Geometry: final body of the model. Coordinates: model frame, mm. Face numbers are marked on the shaded views. A direction names the side the tool comes from. Give positions to 0.01 mm unless a question says otherwise; leave off trailing zeros. Order: outer loops, then holes, each group sorted by start corner. A loop starts at its lowest first (then second) coordinate and runs counter-clockwise, first axis right, second up. Notation, with made-up numbers: (32.5, -37.75) - (37.5, -37.75) arc R27 cw to (37.5, -9.75) - close; hole circle Ø7 at (-5.5, -24.5). An arc over 180 degrees is marked (long way). Write item = value, one per line. Start each with the question number.
from build123d import *

# Parameters (mm, degrees)
SKETCH1_W                      = 15.5
SKETCH1_H                      = 19.5
SKETCH1_W_2                    = 9.9
SKETCH1_H_2                    = 13.9
BOSS_EXTRUDE1_DEPTH            = 4.05
SKETCH2_W                      = 19.5
SKETCH2_H                      = 9
SKETCH2_R                      = 1.5
BOSS_EXTRUDE2_DEPTH            = 2.8
CHAMFER1_SIZE                  = 2.5
FILLET1_R                      = 2
FILLET2_R                      = 0.5
CHAMFER2_SIZE                  = 0.5
CUT_EXTRUDE1_DEPTH             = 1.0000001
CUT_EXTRUDE1_DIRECTION_2_REACH = 17.5


with BuildPart() as part:
    # Sketch1 → Boss-Extrude1 (new body, symmetric)
    with BuildSketch(Plane(origin=(0, 0, 0), x_dir=(1, 0, 0), z_dir=(0, 1, 0))):
        Rectangle(SKETCH1_W, SKETCH1_H)
        Rectangle(SKETCH1_W_2, SKETCH1_H_2, mode=Mode.SUBTRACT)
    extrude(amount=BOSS_EXTRUDE1_DEPTH, both=True)

    # Sketch2 → Boss-Extrude2 (add)
    with BuildSketch(Plane.ZY.offset(7.75)):
        with Locations((0, -8.55)):
            Rectangle(SKETCH2_W, SKETCH2_H)
        with Locations((-5.25, -8.55)):
            Circle(SKETCH2_R, mode=Mode.SUBTRACT)
        with Locations((5.25, -8.55)):
            Circle(SKETCH2_R, mode=Mode.SUBTRACT)
    extrude(amount=-BOSS_EXTRUDE2_DEPTH)

    # Chamfer1
    chamfer1_edges = [part.edges().sort_by_distance(p)[0] for p in [
        (-4.95, -4.05, -8.35),
        (-4.95, -4.05, 8.35),
    ]]
    chamfer(chamfer1_edges, length=CHAMFER1_SIZE)

    # Fillet1
    fillet1_edges = [part.edges().sort_by_distance(p)[0] for p in [
        (-7.75, -4.5, -9.75),
        (7.75, 0, -9.75),
        (7.75, 0, 9.75),
        (-7.75, -4.5, 9.75),
    ]]
    fillet(fillet1_edges, radius=FILLET1_R)

    # Fillet2
    fillet2_edges = [part.edges().sort_by_distance(p)[0] for p in [
        (4.95, -4.05, 0),
        (1.25, -4.05, -6.95),
        (-4.95, 4.05, 0),
        (0, 4.05, 6.95),
        (4.95, 4.05, 0),
        (0, 4.05, -6.95),
        (-5.35, -13.05, -9.75),
        (-4.95, -9.8, 9.75),
        (-4.95, -13.05, 0),
        (-5.35, -13.05, 9.75),
        (1.65, -4.05, 9.75),
        (1.25, -4.05, 6.95),
        (-2.45, -4.05, 8.35),
        (-2.45, -4.05, -8.35),
        (-4.95, -9.8, -9.75),
        (-3.7, -5.3, -9.75),
        (-3.7, -5.3, -6.95),
        (-3.7, -5.3, 6.95),
        (-3.7, -5.3, 9.75),
        (1.65, -4.05, -9.75),
        (0, 4.05, -9.75),
        (7.75, -4.05, 0),
        (7.164213562, -4.05, 9.164213562),
        (7.164213562, -4.05, -9.164213562),
        (7.75, 4.05, 0),
        (-7.75, 4.05, 0),
        (0, 4.05, 9.75),
        (-7.164213562, 4.05, 9.164213562),
        (-7.164213562, 4.05, -9.164213562),
        (7.164213562, 4.05, 9.164213562),
        (7.164213562, 4.05, -9.164213562),
        (-7.75, -13.05, 0),
        (-7.164213562, -13.05, 9.164213562),
        (-7.164213562, -13.05, -9.164213562),
    ]]
    fillet(fillet2_edges, radius=FILLET2_R)

    # Chamfer2
    chamfer2_edges = [part.edges().sort_by_distance(p)[0] for p in [
        (-4.95, -8.55, 3.75),
        (-4.95, -8.55, -6.75),
    ]]
    chamfer(chamfer2_edges, length=CHAMFER2_SIZE)

    # Sketch3 → Cut-Extrude1 (cut)
    with BuildSketch(Plane.ZY.offset(7.75)):
        with BuildLine():
            Line((-3.5, 0.55), (3.5, 0.55))
            ThreePointArc((3.5, 0.55), (3.853553391, 0.403553391), (4, 0.05))
            Line((4, 0.05), (4, -2.22))
            ThreePointArc((4, -2.22), (3.853553391, -2.573553391), (3.5, -2.72))
            Line((3.5, -2.72), (-3.5, -2.72))
            ThreePointArc((-3.5, -2.72), (-3.853553391, -2.573553391), (-4, -2.22))
            Line((-4, -2.22), (-4, 0.05))
            ThreePointArc((-4, 0.05), (-3.853553391, 0.403553391), (-3.5, 0.55))
        make_face()
    extrude(amount=CUT_EXTRUDE1_DEPTH, mode=Mode.SUBTRACT)

    # Sketch3 → Cut-Extrude1 direction 2 (cut, up to next)
    with BuildSketch(Plane.ZY.offset(7.75), mode=Mode.PRIVATE) as cut_extrude1_direction_2_sk1:
        with BuildLine():
            Line((-3.5, 0.55), (3.5, 0.55))
            ThreePointArc((3.5, 0.55), (3.853553391, 0.403553391), (4, 0.05))
            Line((4, 0.05), (4, -2.22))
            ThreePointArc((4, -2.22), (3.853553391, -2.573553391), (3.5, -2.72))
            Line((3.5, -2.72), (-3.5, -2.72))
            ThreePointArc((-3.5, -2.72), (-3.853553391, -2.573553391), (-4, -2.22))
            Line((-4, -2.22), (-4, 0.05))
            ThreePointArc((-4, 0.05), (-3.853553391, 0.403553391), (-3.5, 0.55))
        make_face()
    cut_extrude1_direction_2_tool1 = extrude(cut_extrude1_direction_2_sk1.sketch, amount=-CUT_EXTRUDE1_DIRECTION_2_REACH, mode=Mode.PRIVATE) & part.part
    add(cut_extrude1_direction_2_tool1.solids().sort_by_distance((-7.75, -1.085, 0))[0], mode=Mode.SUBTRACT)


solid = part.part
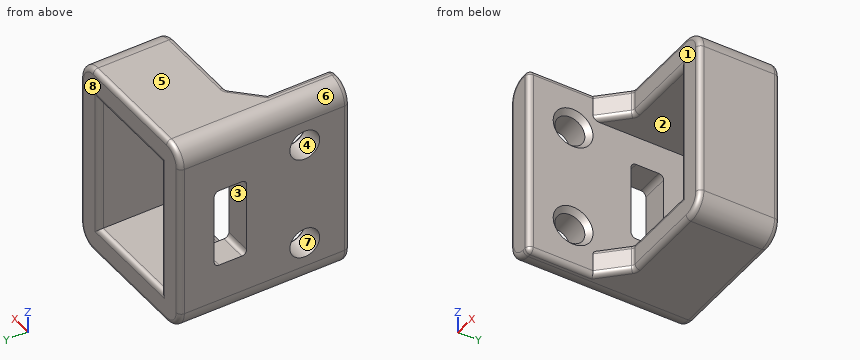
Q1. Pull-direction query (Y, two-part tool) for the marked faces 6, 7 and 8; classes: +Y half, -Y half, draft (parallel to the pull), parting line (faces both ways), or undercut.
Q2. Section B-B, the plane z = -0.5. Return the cut outline in (x, y).
Q3. Contact query for flat-ended pins moving along their axis: pin 1 (7.5 mm diameter, centred on x = 1.5, z = -3, fed in from -Y); pin 2 (0.7 mm diameter, centred on x = -7, y = -0.5, fed in from -Z). Output: stop coordinate, or through.
Q4. Material intervals for line 1 along Z through (x, y) = (1.5, 2.25); line 2 along Y through (x, z) = (-6.9, 5.25), sorted ascending. Write a range as from..to.
Q5. Section C-C, the plane y = -8.55. Return the cut outline in (x, z).
Q6. Set-up query: the marked faces 1, 2, 3, 4 and 5. Return all of +Z, -Z, +X, -X, +Y, -Y with unobstructed straight access to the full face (end or side cutting, diameter ignored); none if empty.
Q7. Section D-D, the plane z = 5.25. Return the cut outline in (x, y).
Q8. Section A-A, the plane x = 0.5. Return the cut outline in (y, z), then the cut area to 3 significant figures.
The answers:
q1.face_6 = draft
q1.face_7 = undercut
q1.face_8 = +Y half
q2.outline = (-7.75, -12.55) arc R0.5 ccw to (-7.25, -13.05) - (-5.45, -13.05) arc R0.5 ccw to (-4.95, -12.55) - (-4.95, -2.72) - (-7.75, -2.72) - close; (-7.75, 0.55) - (-4.95, 0.55) - (-4.95, 3.55) arc R0.5 ccw to (-5.45, 4.05) - (-7.25, 4.05) arc R0.5 ccw to (-7.75, 3.55) - close; (4.95, -3.55) arc R0.5 ccw to (5.45, -4.05) - (7.25, -4.05) arc R0.5 ccw to (7.75, -3.55) - (7.75, 3.55) arc R0.5 ccw to (7.25, 4.05) - (5.45, 4.05) arc R0.5 ccw to (4.95, 3.55) - close
q3.pin_1 = -4.01
q3.pin_2 = -9.54
q4.line_1 = -9.75..-6.95, 6.95..9.75
q4.line_2 = -13.05..-10.05, -7.05..4.05
q5.outline = (-7.75, -7.75) arc R2 ccw to (-5.75, -9.75) - (-5.45, -9.75) arc R0.5 ccw to (-4.95, -9.25) - (-4.95, -7.25) - (-5.45, -6.75) - (-7.75, -6.75) - close; (-7.75, -3.75) - (-5.45, -3.75) - (-4.95, -3.25) - (-4.95, 3.25) - (-5.45, 3.75) - (-7.75, 3.75) - close; (-7.75, 6.75) - (-5.45, 6.75) - (-4.95, 7.25) - (-4.95, 9.25) arc R0.5 ccw to (-5.45, 9.75) - (-5.75, 9.75) arc R2 ccw to (-7.75, 7.75) - close
q6.face_1 = +Z, -Z, +X, -Y
q6.face_2 = +Y, -Y
q6.face_3 = -X
q6.face_4 = +X, -X
q6.face_5 = +Z, +X, -X, +Y, -Y
q7.outline = (-7.75, -12.55) arc R0.5 ccw to (-7.25, -13.05) - (-5.45, -13.05) arc R0.5 ccw to (-4.95, -12.55) - (-4.95, -10.55) - (-5.45, -10.05) - (-7.75, -10.05) - close; (-7.75, -7.05) - (-5.45, -7.05) - (-4.95, -6.55) - (-4.95, 3.55) arc R0.5 ccw to (-5.45, 4.05) - (-7.25, 4.05) arc R0.5 ccw to (-7.75, 3.55) - close; (4.95, -3.55) arc R0.5 ccw to (5.45, -4.05) - (7.25, -4.05) arc R0.5 ccw to (7.75, -3.55) - (7.75, 3.55) arc R0.5 ccw to (7.25, 4.05) - (5.45, 4.05) arc R0.5 ccw to (4.95, 3.55) - close
q8.outline = (-4.05, -9.25) arc R0.5 ccw to (-3.55, -9.75) - (3.55, -9.75) arc R0.5 ccw to (4.05, -9.25) - (4.05, -7.45) arc R0.5 ccw to (3.55, -6.95) - (-3.55, -6.95) arc R0.5 ccw to (-4.05, -7.45) - close; (-4.05, 7.45) arc R0.5 ccw to (-3.55, 6.95) - (3.55, 6.95) arc R0.5 ccw to (4.05, 7.45) - (4.05, 9.25) arc R0.5 ccw to (3.55, 9.75) - (-3.55, 9.75) arc R0.5 ccw to (-4.05, 9.25) - close
q8.area = 44.9 mm²
